Autodesk Inventor part; units mm, degrees
ref_plane "YZ Plane" through (0, 0, 0) normal (1, 0, 0) x (0, 1, 0)
ref_plane "XZ Plane" through (0, 0, 0) normal (0, 1, 0) x (-1, 0, 0)
ref_plane "XY Plane" through (0, 0, 0) normal (0, 0, 1) x (1, 0, 0)
sketch "Sketch1" plane through (0, 0, 0) normal (0, 0, 1) x (1, 0, 0)
  line L0 (-32.5, 75) -> (32.5, 75)
  line L1 (32.5, 75) -> (32.5, -60)
  line L2 (32.5, -60) -> (-32.5, -60)
  line L3 (-32.5, -60) -> (-32.5, 75)
  point P0 (0, 0)
  dimension "d0" = 65
  dimension "d1" = 135
  dimension "d2" = 32.5
  dimension "d3" = 60
extrude "Extrusion1" add sketch "Sketch1" along normal blind 5
sketch "Sketch2" plane through (0, 0, 5) normal (0, 0, 1) x (1, 0, 0)
  line L0 (-32.5, 75) -> (-32.5, -60)
  line L1 (-32.5, -60) -> (32.5, -60)
  line L2 (-32.5, -56) -> (32.5, -56)
  line L3 (32.5, -56) -> (32.5, -60)
  line L4 (32.5, -60) -> (-32.5, -60)
  line L5 (-32.5, -60) -> (-32.5, -56)
  point P0 (0, 0)
  dimension "d6" = 4
extrude "Extrusion2" add sketch "Sketch2" along normal blind 8
sketch "Sketch3" plane through (0, 0, 13) normal (0, 0, 1) x (1, 0, 0)
  line L0 (-32.5, -60) -> (-32.5, 75)
  line L1 (32.5, 75) -> (32.5, -60)
  line L2 (-32.5, -50) -> (32.5, -50)
  line L3 (32.5, -50) -> (32.5, -60)
  line L4 (32.5, -60) -> (-32.5, -60)
  line L5 (-32.5, -60) -> (-32.5, -50)
  point P0 (0, 0)
  dimension "d9" = 10
extrude "Extrusion3" add sketch "Sketch3" along normal blind 4
sketch "Sketch4" plane through (0, 0, 5) normal (0, 0, 1) x (1, 0, 0)
  line L0 (-32.5, -60) -> (-32.5, 75)
  line L1 (32.5, 75) -> (32.5, -60)
  line L2 (32.5, 75) -> (32.5, 71)
  line L3 (-32.5, 71) -> (-32.5, 75)
  point P0 (0, 0)
sketch "Sketch6" plane through (-32.5, -60, 0) normal (0, -1, 0) x (1, 0, 0)
  line L0 (65, 13) -> (0, 13)
  line L1 (21.6667, 13) -> (43.3333, 13)
  line L2 (43.3333, 13) -> (43.3333, 5.6667)
  line L3 (43.3333, 5.6667) -> (21.6667, 5.6667)
  line L4 (21.6667, 5.6667) -> (21.6667, 13)
  line L5 (65, 0) -> (65, 17)
  line L6 (0, 0) -> (0, 17)
  line L7 (65, 0) -> (0, 0)
  line L8 (0, 17) -> (65, 17)
  point P0 (32.5, 0)
  dimension "d18" = 21.6667
  dimension "d19" = 21.6667
  dimension "d20" = 5.6667
  dimension "d21" = 4
extrude "Extrusion6" cut sketch "Sketch6" against normal blind 206 contours L2 L3 L4 L0
sketch "Sketch7" plane through (0, 0, 0) normal (0, 0, -1) x (-1, 0, 0)
  line L0 (32.5, -56) -> (-32.5, -56)
  line L1 (29.5, -56) -> (-29.5, -56)
  line L2 (-29.5, -56) -> (-29.5, -50)
  line L3 (-32.5, -50) -> (32.5, -50)
  line L4 (-29.5, -50) -> (29.5, -50)
  line L5 (29.5, -50) -> (29.5, -56)
  line L6 (32.5, -60) -> (32.5, 75)
  line L7 (-32.5, 75) -> (-32.5, -60)
  line L8 (29.5, -46) -> (-29.5, -46)
  line L9 (-29.5, -46) -> (-29.5, -40)
  line L10 (-29.5, -40) -> (29.5, -40)
  line L11 (29.5, -40) -> (29.5, -46)
  line L12 (29.5, -36) -> (-29.5, -36)
  line L13 (-29.5, -36) -> (-29.5, -30)
  line L14 (-29.5, -30) -> (29.5, -30)
  line L15 (29.5, -30) -> (29.5, -36)
  line L16 (29.5, -26) -> (-29.5, -26)
  line L17 (-29.5, -26) -> (-29.5, -20)
  line L18 (-29.5, -20) -> (29.5, -20)
  line L19 (29.5, -20) -> (29.5, -26)
  line L20 (29.5, -16) -> (-29.5, -16)
  line L21 (-29.5, -16) -> (-29.5, -10)
  line L22 (-29.5, -10) -> (29.5, -10)
  line L23 (29.5, -10) -> (29.5, -16)
  line L24 (32.5, 65) -> (-32.5, 65)
  line L25 (-32.5, 71) -> (32.5, 71)
  line L26 (29.5, 65) -> (-29.5, 65)
  line L27 (-29.5, 65) -> (-29.5, 71)
  line L28 (-29.5, 71) -> (29.5, 71)
  line L29 (29.5, 71) -> (29.5, 65)
  line L30 (29.5, 51.5) -> (-29.5, 51.5)
  line L31 (29.5, 57.5) -> (29.5, 51.5)
  line L32 (-29.5, 57.5) -> (29.5, 57.5)
  line L33 (-29.5, 51.5) -> (-29.5, 57.5)
  line L34 (29.5, 38) -> (-29.5, 38)
  line L35 (29.5, 44) -> (29.5, 38)
  line L36 (-29.5, 44) -> (29.5, 44)
  line L37 (-29.5, 38) -> (-29.5, 44)
  line L38 (29.5, 24.5) -> (-29.5, 24.5)
  line L39 (29.5, 30.5) -> (29.5, 24.5)
  line L40 (-29.5, 30.5) -> (29.5, 30.5)
  line L41 (-29.5, 24.5) -> (-29.5, 30.5)
  line L42 (29.5, 11) -> (-29.5, 11)
  line L43 (29.5, 17) -> (29.5, 11)
  line L44 (-29.5, 17) -> (29.5, 17)
  line L45 (-29.5, 11) -> (-29.5, 17)
  point P0 (0, 0)
  dimension "d24" = 3
  dimension "d25" = 3
  dimension "d30" = 10
  dimension "d35" = 3
  dimension "d36" = 3
  dimension "d39" = 13.5
extrude "Extrusion7" cut sketch "Sketch7" against normal up to surface (5 mm away) contours L0 L2 L3 L5
extrude "Extrusion8" cut sketch "Sketch7" against normal up to surface (5 mm away) contours L24 L27 L25 L29 | L8 L9 L10 L11 | L12 L13 L14 L15 | L16 L17 L18 L19 | L20 L21 L22 L23 | L30 L33 L32 L31 | L34 L37 L36 L35 | L38 L41 L40 L39 | L42 L45 L44 L43
sketch "Sketch8" plane through (0, 0, 0) normal (0, 0, -1) x (-1, 0, 0)
  line L0 (32.5, 75) -> (-32.5, 75)
  line L1 (-29.5, 11) -> (29.5, 11)
  line L2 (-3, 75) -> (3, 75)
  line L3 (3, 75) -> (3, 11)
  line L4 (3, 11) -> (-3, 11)
  line L5 (-3, 11) -> (-3, 75)
  line L6 (32.5, -60) -> (32.5, 75)
  line L7 (-32.5, 75) -> (-32.5, -60)
  point P0 (0, 0)
  dimension "d46" = 29.5
  dimension "d47" = 29.5
extrude "Extrusion9" cut sketch "Sketch8" against normal blind 206
properties part number "Kirtiman phone charger design"
Part model, mm, in its own coordinate system. A direction names the side the tool comes from. Round coordinates to 2 decimals unless told otherwise and drop trailing zeros. Loops run counter-clockwise (first coordinate to the right, second up) from the corner with the lowest first, then second, coordinate; pieces in that order, holes last. Notation, with made-up numbers: (61, 23.25) -> (110, 23.25) arc R10 ccw to (110, 33.25) -> close; hole circle Ø5 at (-12.5, -22.5). An arc over 180 degrees is marked (long way). Use a Markdown table: item, result.
1) Cut at C-C, the plane x = -4.5. State how many separate pieces and enclosed holes the cut face has, and give its area (3 significant figures).
The answers:
| item | result |
|---|---|
| separate pieces | 12 |
| enclosed holes | 0 |
| area | 418 mm2 |
2) Probe line 1 (X direction, y = 44.5, z = 2.75); line 2 (Y direction, x = 19.5, z = 15.75); line 3 (Z direction, x = 15.5, y = -52.5). List the from-to ranges inside material, lowest first. Write a range as [from, to].
The answers:
| item | result |
|---|---|
| line 1 | x = [-32.5, -3], [3, 32.5] |
| line 2 | y = [-60, -50] |
| line 3 | z = [13, 17] |
3) Cut at B-B, the plane z = 11.25. List the corners of the cut face in (x, y).
The answers:
| item | result |
|---|---|
| outline | (-32.5, -60) -> (-10.83, -60) -> (-10.83, -56) -> (-32.5, -56) -> close; (10.83, -60) -> (32.5, -60) -> (32.5, -56) -> (10.83, -56) -> close |
4) Drop a flat-ended pin along its axis: pin 1 Ø5 at (x, y) = (26, 51.5) entering from +Z. Give the stop position or say it passes through.
The answers:
| item | result |
|---|---|
| pin 1 | stops at z = 5 |
5) Pull direction Z, two halves, no side cores. Call faces 3 (the flat face through (0, -55, 17)), 4 (the flat face through (0, -54, 13)), 5 (the flat face through (-3, 73, 2)): pulls with the +Z half, pulls with the -Z half, needs draft (parallel to the pull), parting line crosses it, or undercut.
The answers:
| item | result |
|---|---|
| face 3 | pulls with the +Z half |
| face 4 | undercut |
| face 5 | needs draft |
6) Cut at A-A, the plane y = 28. List the corners of the cut face in (x, z).
The answers:
| item | result |
|---|---|
| outline | (-32.5, 0) -> (-29.5, 0) -> (-29.5, 5) -> (-32.5, 5) -> close; (29.5, 0) -> (32.5, 0) -> (32.5, 5) -> (29.5, 5) -> close |
7) Tool access for faces 1 (the flat face through (32.5, 3, 4)), 2 (the flat face through (16, 51.5, 2)): list every direction of +Z, -Z, +X, -X, +Y, -Y with a clear straight run to the whole face (end or side of a thin tool).
The answers:
| item | result |
|---|---|
| face 1 | +Z, -Z, +X, +Y, -Y |
| face 2 | +Z, -Z |
